Read the model definition and answer for the solid it produces. Units are mm, in the model's axes. A direction names the side the tool comes from. Round coordinates to 2 decimals unless told otherwise and drop trailing zeros. Loops run counter-clockwise (first coordinate to the right, second up) from the corner with the lowest first, then second, coordinate; pieces in that order, holes last. Notation, with made-up numbers: (-10.75, 20.5) -> (46.25, 20.5) arc R30 cw to (46.25, 47.5) -> close; hole circle Ø4 at (57.5, -36.5). An arc over 180 degrees is marked (long way). Put each result on its own line as item: value.
from build123d import *

# Parameters (mm, degrees)
ESBO_O1_R                = 1.6
ESBO_O1_R_2              = 3
ESBO_O1_R_3              = 12
ESBO_O1_R_4              = 3.5
ESBO_O1_R_5              = 3.05
RESSALTO_EXTRUS_O1_DEPTH = 6
ESBO_O2_R                = 3
CORTE_EXTRUS_O1_DEPTH    = 10


with BuildPart() as part:
    # Esboço1 → Ressalto-extrusão1 (new body)
    with BuildSketch(Plane(origin=(0, 0, 0), x_dir=(1, 0, 0), z_dir=(0, 1, 0))):
        with BuildLine():
            Line((-80.557360207, -153.648697641), (51.472077044, -153.648697641))
            ThreePointArc((51.472077044, -153.648697641), (53.593397388, -152.770017984), (54.472077044, -150.648697641))
            Line((54.472077044, -150.648697641), (54.472077044, -60.788592817))
            ThreePointArc((54.472077044, -60.788592817), (57.401009232, -53.717525005), (64.472077044, -50.788592817))
            Line((64.472077044, -50.788592817), (178.527922956, -50.788592817))
            ThreePointArc((178.527922956, -50.788592817), (185.598990768, -47.859660628), (188.527922956, -40.788592817))
            Line((188.527922956, -40.788592817), (188.527922956, 28))
            ThreePointArc((188.527922956, 28), (185.01320433, 36.485281374), (176.527922956, 40))
            Line((176.527922956, 40), (-176.527922956, 40))
            ThreePointArc((-176.527922956, 40), (-185.01320433, 36.485281374), (-188.527922956, 28))
            Line((-188.527922956, 28), (-188.527922956, -45.678134892))
            ThreePointArc((-188.527922956, -45.678134892), (-187.614477346, -50.270336081), (-185.01320433, -54.163416267))
            Line((-185.01320433, -54.163416267), (-89.042641582, -150.133979015))
            ThreePointArc((-89.042641582, -150.133979015), (-85.149561396, -152.735252031), (-80.557360207, -153.648697641))
        make_face()
        with Locations(Location((-81.027922956, -58.148697641, 0), (0, 0, 90))):
            Circle(ESBO_O1_R, mode=Mode.SUBTRACT)
        with Locations(Location((-81.027922956, -146.148697641, 0), (0, 0, 90))):
            Circle(ESBO_O1_R, mode=Mode.SUBTRACT)
        with Locations(Location((46.972077044, -58.148697641, 0), (0, 0, 90))):
            Circle(ESBO_O1_R, mode=Mode.SUBTRACT)
        with Locations(Location((46.972077044, -146.148697641, 0), (0, 0, 90))):
            Circle(ESBO_O1_R, mode=Mode.SUBTRACT)
        with Locations(Location((176.311042956, -38.431817641, 0), (0, 0, 90))):
            Circle(ESBO_O1_R_2, mode=Mode.SUBTRACT)
        with Locations(Location((0, -38.431817641, 0), (0, 0, 90))):
            Circle(ESBO_O1_R_2, mode=Mode.SUBTRACT)
        with Locations(Location((-140.527922956, 10, 0), (0, 0, 90))):
            Circle(ESBO_O1_R_3, mode=Mode.SUBTRACT)
        with Locations(Location((-140.527922956, -6, 0), (0, 0, 270))):
            Circle(ESBO_O1_R, mode=Mode.SUBTRACT)
        with Locations(Location((-154.384329416, 2, 0), (0, 0, 270))):
            Circle(ESBO_O1_R, mode=Mode.SUBTRACT)
        with Locations(Location((-154.384329416, 18, 0), (0, 0, 270))):
            Circle(ESBO_O1_R, mode=Mode.SUBTRACT)
        with Locations(Location((-84.367438628, 32.5, 0), (0, 0, 90))):
            Circle(ESBO_O1_R_2, mode=Mode.SUBTRACT)
        with Locations(Location((-176.311042956, -38.431817641, 0), (0, 0, 90))):
            Circle(ESBO_O1_R_2, mode=Mode.SUBTRACT)
        with Locations(Location((140.527922956, 10, 0), (0, 0, 90))):
            Circle(ESBO_O1_R_4, mode=Mode.SUBTRACT)
        with Locations(Location((148.527922956, 0, 0), (0, 0, 90))):
            Circle(ESBO_O1_R, mode=Mode.SUBTRACT)
        with Locations(Location((148.527922956, 20, 0), (0, 0, 90))):
            Circle(ESBO_O1_R, mode=Mode.SUBTRACT)
        with Locations(Location((132.527922956, 0, 0), (0, 0, 90))):
            Circle(ESBO_O1_R, mode=Mode.SUBTRACT)
        with Locations(Location((132.527922956, 20, 0), (0, 0, 90))):
            Circle(ESBO_O1_R, mode=Mode.SUBTRACT)
        with Locations(Location((-140.527922956, 26, 0), (0, 0, 270))):
            Circle(ESBO_O1_R, mode=Mode.SUBTRACT)
        with Locations(Location((-126.671516495, 18, 0), (0, 0, 270))):
            Circle(ESBO_O1_R, mode=Mode.SUBTRACT)
        with Locations(Location((-126.671516495, 2, 0), (0, 0, 270))):
            Circle(ESBO_O1_R, mode=Mode.SUBTRACT)
        with Locations(Location((-63.17160518, -16, 0), (0, 0, 270))):
            Circle(ESBO_O1_R, mode=Mode.SUBTRACT)
        with Locations(Location((-77.02801164, -8, 0), (0, 0, 270))):
            Circle(ESBO_O1_R, mode=Mode.SUBTRACT)
        with Locations(Location((-77.02801164, 8, 0), (0, 0, 270))):
            Circle(ESBO_O1_R, mode=Mode.SUBTRACT)
        with Locations(Location((-63.17160518, 16, 0), (0, 0, 270))):
            Circle(ESBO_O1_R, mode=Mode.SUBTRACT)
        with Locations(Location((-49.315198719, 8, 0), (0, 0, 270))):
            Circle(ESBO_O1_R, mode=Mode.SUBTRACT)
        with Locations(Location((-49.315198719, -8, 0), (0, 0, 270))):
            Circle(ESBO_O1_R, mode=Mode.SUBTRACT)
        with Locations(Location((-63.17160518, 0, 0), (0, 0, 270))):
            Circle(ESBO_O1_R_3, mode=Mode.SUBTRACT)
        with Locations(Location((-33.527922956, -20.648697641, 0), (0, 0, 270))):
            Circle(ESBO_O1_R_2, mode=Mode.SUBTRACT)
        with Locations(Location((79.527922956, 10, 0), (0, 0, 270))):
            Circle(ESBO_O1_R_2, mode=Mode.SUBTRACT)
        with Locations(Location((99.722077044, 0, 0), (0, 0, 270))):
            Circle(ESBO_O1_R, mode=Mode.SUBTRACT)
        with Locations(Location((49.222077044, -43, 0), (0, 0, 270))):
            Circle(ESBO_O1_R, mode=Mode.SUBTRACT)
        with Locations(Location((-30.527922956, 6, 0), (0, 0, 270))):
            Circle(ESBO_O1_R, mode=Mode.SUBTRACT)
        with Locations(Location((19.472077044, 6, 0), (0, 0, 270))):
            Circle(ESBO_O1_R, mode=Mode.SUBTRACT)
        with Locations(Location((60.527922956, 6, 0), (0, 0, 270))):
            Circle(ESBO_O1_R, mode=Mode.SUBTRACT)
        with Locations(Location((40.527922956, 6, 0), (0, 0, 270))):
            Circle(ESBO_O1_R, mode=Mode.SUBTRACT)
        with Locations(Location((159.467922956, 24.07, 0), (0, 0, 270))):
            Circle(ESBO_O1_R_5, mode=Mode.SUBTRACT)
        with Locations(Location((159.467922956, -3.93, 0), (0, 0, 270))):
            Circle(ESBO_O1_R_5, mode=Mode.SUBTRACT)
        with Locations(Location((159.467922956, -28.93, 0), (0, 0, 270))):
            Circle(ESBO_O1_R_5, mode=Mode.SUBTRACT)
        with Locations(Location((-178.527922956, 19.5, 0), (0, 0, 270))):
            Circle(ESBO_O1_R_2, mode=Mode.SUBTRACT)
        with Locations(Location((-98.527922956, 19.5, 0), (0, 0, 270))):
            Circle(ESBO_O1_R_2, mode=Mode.SUBTRACT)
        with Locations(Location((57.327922956, 25.68, 0), (0, 0, 270))):
            Circle(ESBO_O1_R_2, mode=Mode.SUBTRACT)
        with BuildLine():
            Line((-122.576844598, -50.788592817), (-93.527922956, -50.788592817))
            ThreePointArc((-93.527922956, -50.788592817), (-89.99238905, -52.253058911), (-88.527922956, -55.788592817))
            Line((-88.527922956, -55.788592817), (-88.527922956, -84.837514459))
            ThreePointArc((-88.527922956, -84.837514459), (-91.614505794, -89.456912121), (-97.063456862, -88.373048365))
            Line((-97.063456862, -88.373048365), (-126.112378504, -59.324126723))
            ThreePointArc((-126.112378504, -59.324126723), (-127.196242261, -53.875175655), (-122.576844598, -50.788592817))
        make_face(mode=Mode.SUBTRACT)
        with BuildLine():
            Line((39.472077044, -60.648697641), (39.472077044, -128.648697641))
            ThreePointArc((39.472077044, -128.648697641), (36.543144856, -135.719765453), (29.472077044, -138.648697641))
            Line((29.472077044, -138.648697641), (-63.527922956, -138.648697641))
            ThreePointArc((-63.527922956, -138.648697641), (-70.598990768, -135.719765453), (-73.527922956, -128.648697641))
            Line((-73.527922956, -128.648697641), (-73.527922956, -60.648697641))
            ThreePointArc((-73.527922956, -60.648697641), (-70.598990768, -53.577629829), (-63.527922956, -50.648697641))
            Line((-63.527922956, -50.648697641), (29.472077044, -50.648697641))
            ThreePointArc((29.472077044, -50.648697641), (36.543144856, -53.577629829), (39.472077044, -60.648697641))
        make_face(mode=Mode.SUBTRACT)
        with BuildLine():
            Line((148.722077044, -43), (148.722077044, -23))
            ThreePointArc((148.722077044, -23), (150.222077044, -21.5), (151.722077044, -23))
            Line((151.722077044, -23), (151.722077044, -43))
            ThreePointArc((151.722077044, -43), (150.222077044, -44.5), (148.722077044, -43))
        make_face(mode=Mode.SUBTRACT)
        with BuildLine():
            Line((133.722077044, -43), (133.722077044, -23))
            ThreePointArc((133.722077044, -23), (132.222077044, -21.5), (130.722077044, -23))
            Line((130.722077044, -23), (130.722077044, -43))
            ThreePointArc((130.722077044, -43), (132.222077044, -44.5), (133.722077044, -43))
        make_face(mode=Mode.SUBTRACT)
        with BuildLine():
            Line((67.977922956, 25), (67.977922956, 35))
            ThreePointArc((67.977922956, 35), (70.527922956, 37.55), (73.077922956, 35))
            Line((73.077922956, 35), (73.077922956, 25))
            ThreePointArc((73.077922956, 25), (70.527922956, 22.45), (67.977922956, 25))
        make_face(mode=Mode.SUBTRACT)
        with BuildLine():
            Line((101.227922956, 25), (101.227922956, 35))
            ThreePointArc((101.227922956, 35), (103.777922956, 37.55), (106.327922956, 35))
            Line((106.327922956, 35), (106.327922956, 25))
            ThreePointArc((106.327922956, 25), (103.777922956, 22.45), (101.227922956, 25))
        make_face(mode=Mode.SUBTRACT)
    extrude(amount=-RESSALTO_EXTRUS_O1_DEPTH)

    # Esboço2 → Corte-extrusão1 (cut)
    with BuildSketch(Plane(origin=(0, 0, 0), x_dir=(1, 0, 0), z_dir=(0, 1, 0))):
        with Locations(Location((-117.838060117, -94.468502794, 0), (0, 0, 270))):
            Circle(ESBO_O2_R)
    extrude(amount=-CORTE_EXTRUS_O1_DEPTH, mode=Mode.SUBTRACT)


solid = part.part
Item 1: The part is cut by section A-A (x = -20). Determine the outline of the cut face in (y, z).
Derived:
outline: (-6, -40) -> (0, -40) -> (0, 50.65) -> (-6, 50.65) -> close; (-6, 138.65) -> (0, 138.65) -> (0, 153.65) -> (-6, 153.65) -> close
Item 2: Find the intervals of material crossed by line 1 along Z through (x, y) = (-53, -1.55); line 2 along X through (y, z) = (-2.85, -20); line 3 along Z through (x, y) = (61, -4.5), in increasing order.
Derived:
line 1: z = -40 to -6.37, 6.37 to 50.65, 138.65 to 153.65
line 2: x = -188.53 to -181.49, -175.57 to -147.16, -133.89 to -101.49, -95.57 to 130.93, 134.13 to 146.93, 150.13 to 188.53
line 3: z = -40 to -7.53, -4.47 to 51.41
Item 3: The part is cut by section C-C (y = -2.6). State how many separate pieces and enclosed holes the cut face has, then the cut area to 3 significant figures.
Derived:
separate pieces: 1
enclosed holes: 48
area: 41,200 mm^2
Item 4: For a pull along X with two mould halves and no side action, classify faces 3 (the flat face through (-3, -6, 34)), 4 (the flat face through (-137.7, -2.958, 101.477)), 5 (the cylindrical face through (36.465, -2.958, 53.5)) as pulls with the +X half, pulls with the -X half, needs draft (parallel to the pull), parting line crosses it, or undercut.
Derived:
face 3: needs draft
face 4: pulls with the -X half
face 5: undercut
Item 5: Flat-ended cylindrical pins translate along their axes: pin 1 Ø1.5 at (y, z) = (-1.5, 134) entering from +X; pin 2 Ø1 at (x, y) = (-90.5, -3) entering from +Z; pin 3 Ø1.5 at (x, y) = (136, -2) entering from +Z. Find the tip coordinate at first contact, or state that the pin passes through.
Derived:
pin 1: stops at x = 54.47
pin 2: stops at z = 149.18
pin 3: stops at z = 50.79
Item 6: Which of the six approach directions +Z, -Z, +X, -X, +Y, -Y give full straight-line access (tool end or side, diameter ignored) to faces 1 (the cylindrical face through (185.1, -3, -36.4)), 2 (the cylindrical face through (-70.52, -2.96, 135.8))?
Derived:
face 1: -Z, +X, +Y, -Y
face 2: +Y, -Y
Item 7: The part is cut by section B-B (z = 117.5). Determine the outline of the cut face in (x, y), then the cut area to 3 significant figures.
Derived:
outline: (-121.68, -6) -> (-73.53, -6) -> (-73.53, 0) -> (-121.68, 0) -> close; (39.47, -6) -> (54.47, -6) -> (54.47, 0) -> (39.47, 0) -> close
area: 379 mm^2
